Geometry: see drawing. Coordinates: mm, zero at the bounding-box minimum. Round coordinates to 2 decimals unless told otherwise and drop trailing zeros. Loops run counter-clockwise (first coordinate to the right, second up) from the corner with the lowest first, then second, coordinate; pieces in that order, holes last. Notation, with made-up numbers: M 34.5,84 L 91.5,84 A25 cw 91.5,99 Z; hole C 41.5,46 d1. An arc over 180 degrees is marked long. Answer as a JSON object with one key per item and string values.
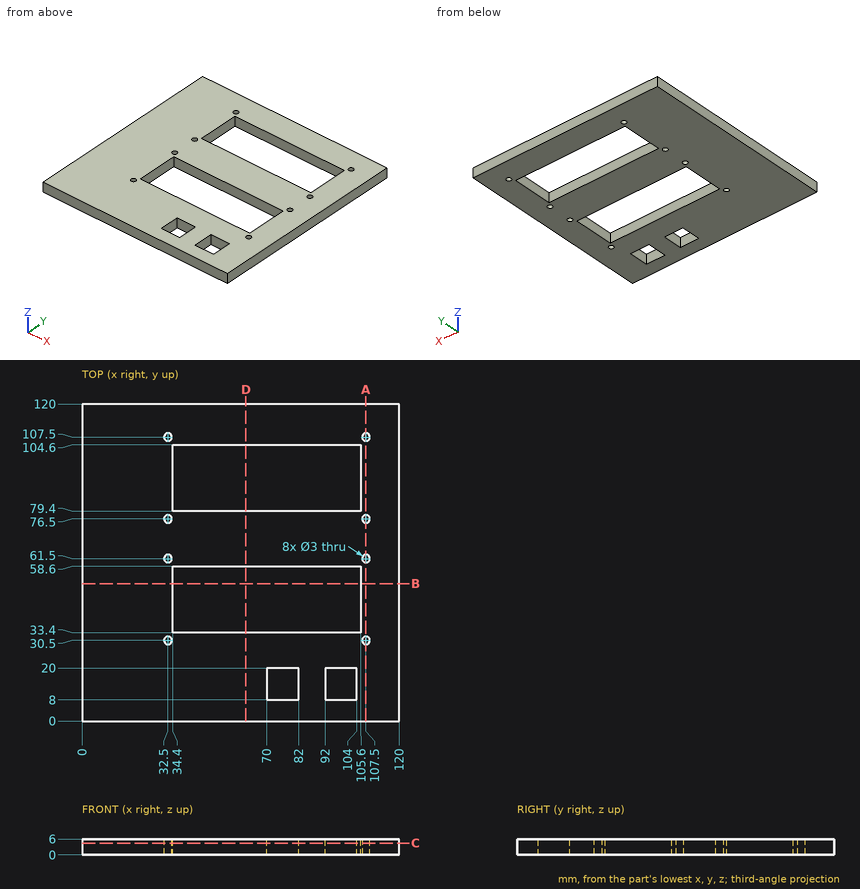
1) Section query C-C (z = 4.4). Count the separate pieces of the cut face and the enclosed holes in it, and give its area (3 significant figures).
Results:
{"separate pieces": "1", "enclosed holes": "12", "area": "10,500 mm2"}
2) Section query D-D (x = 62). Return the cut outline in (y, z).
Results:
{"outline": "M 0,0 L 33.4,0 L 33.4,6 L 0,6 Z; M 58.6,0 L 79.4,0 L 79.4,6 L 58.6,6 Z; M 104.6,0 L 120,0 L 120,6 L 104.6,6 Z"}
3) Section query A-A (x = 107.5). Return the cut outline in (y, z), and give its area (3 significant figures).
Results:
{"outline": "M 0,0 L 29,0 L 29,6 L 0,6 Z; M 32,0 L 60,0 L 60,6 L 32,6 Z; M 63,0 L 75,0 L 75,6 L 63,6 Z; M 78,0 L 106,0 L 106,6 L 78,6 Z; M 109,0 L 120,0 L 120,6 L 109,6 Z", "area": "648 mm2"}
4) Ray query, line 1 (Y direction, x = 91, z = 2.35); line 2 (Y direction, x = 98, z = 3); line 3 (Y direction, x = 107.5, z = 3.3). Return the intervals inside material, ascending.
Results:
{"line 1": "0 to 33.4, 58.6 to 79.4, 104.6 to 120", "line 2": "0 to 8, 20 to 33.4, 58.6 to 79.4, 104.6 to 120", "line 3": "0 to 29, 32 to 60, 63 to 75, 78 to 106, 109 to 120"}
5) Section query B-B (y = 52). Return the cut outline in (x, z).
Results:
{"outline": "M 0,0 L 34.4,0 L 34.4,6 L 0,6 Z; M 105.6,0 L 120,0 L 120,6 L 105.6,6 Z"}
6) Pin query (flat end, axial travel): P1, Ø1.8, axis at x = 107.5, y = 107.5, coming from the +Z side; P2, Ø4, axis at x = 32.5, y = 76.5, coming from the -Z side. Return the tip coordinate at first contact, or that it passes through.
Results:
{"P1": "through", "P2": "z = 0"}
